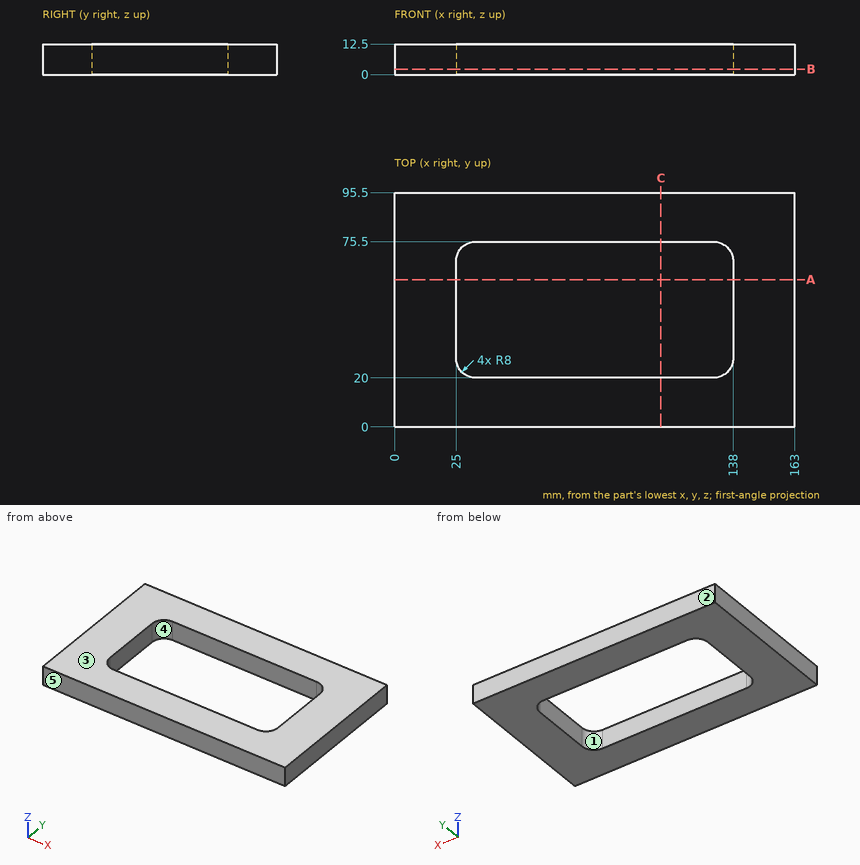
Part print with two shaded views. Sizes in mm from the minimum x, y, z corner. A direction names the side the tool comes from. Round coordinates to 2 decimals unless told otherwise and drop trailing zeros. Loops run counter-clockwise (first coordinate to the right, second up) from the corner with the lowest first, then second, coordinate; pieces in that order, holes last.
1. Slice it at A-A (y = 60). Give the cut face in (x, z).
Solutions:
outline: (0, 0) - (25, 0) - (25, 12.5) - (0, 12.5) - close; (138, 0) - (163, 0) - (163, 12.5) - (138, 12.5) - close
2. Slice it at B-B (z = 2.25). Give the cut face in (x, y).
Solutions:
outline: (0, 0) - (163, 0) - (163, 95.5) - (0, 95.5) - close; hole (25, 28) arc R8 ccw to (33, 20) - (130, 20) arc R8 ccw to (138, 28) - (138, 67.5) arc R8 ccw to (130, 75.5) - (33, 75.5) arc R8 ccw to (25, 67.5) - close
3. Two-plate mould, pull along Y, no slides. Class the marked faces 1, 2 and 3: pulls with the +Y half, pulls with the -Y half, needs draft (parallel to the pull), parting line crosses it, or undercut.
Solutions:
face 1: undercut
face 2: pulls with the +Y half
face 3: needs draft
4. 3-axis set-ups, long thin cutter, end or side, ignore diameter. For the marked faces 4 and 5: which of +Z, -Z, +X, -X, +Y, -Y reach the whole face in a straight line?
Solutions:
face 4: +Z, -Z
face 5: +Z, -Z, +X, -X, -Y
5. Slice it at C-C (x = 108.5). Give the cut face in (y, z).
Solutions:
outline: (0, 0) - (20, 0) - (20, 12.5) - (0, 12.5) - close; (75.5, 0) - (95.5, 0) - (95.5, 12.5) - (75.5, 12.5) - close
6. Drill centre lines: line 1 along X through (y, z) = (42, 2.75); line 2 along Y through (x, z) = (45, 9.75); line 3 along Y through (x, z) = (27.5, 9.25). Where is each one in solid material? Low to high.
Solutions:
line 1: x = 0 to 25, 138 to 163
line 2: y = 0 to 20, 75.5 to 95.5
line 3: y = 0 to 22.19, 73.31 to 95.5
